```python
from build123d import *

# Parameters (mm, degrees)
SKETCH_1_R          = 2.2
SKETCH_1_R_2        = 1.95
SKETCH_1_W          = 40
SKETCH_1_H          = 20
SKETCH_1_W_2        = 16
EXTRUDE_1_DEPTH     = 1.5
SKETCH_2_W          = 120
SKETCH_2_H          = 3
EXTRUDE_2_DEPTH     = 6
SKETCH_3_R          = 2
CUT_EXTRUDE_1_DEPTH = 6


with BuildPart() as part:
    # 草图1 → 凸台-拉伸1 (new, symmetric)
    with BuildSketch(Plane.XY):
        Polygon((-0.084238348, 32.688738727), (91.943563532, 32.688738727), (91.943563532, -45.349139123), (-38.396296283, -45.349139123), (-38.396296283, -11.277844067), (-17.084238348, -11.277844067), (-0.084238348, -11.277844067), (-0.084238348, 8.722155933), align=None)
        with Locations((14.641461985, 3.722155933)):
            Circle(SKETCH_1_R, mode=Mode.SUBTRACT)
        with Locations((14.641461985, -6.277844067)):
            Circle(SKETCH_1_R, mode=Mode.SUBTRACT)
        with Locations((63.041461985, 3.722155933)):
            Circle(SKETCH_1_R, mode=Mode.SUBTRACT)
        with Locations((63.041461985, -6.277844067)):
            Circle(SKETCH_1_R, mode=Mode.SUBTRACT)
        with Locations((68.719491165, 27.139714958)):
            Circle(SKETCH_1_R_2, mode=Mode.SUBTRACT)
        with Locations((38.841461985, -1.277844067)):
            Rectangle(SKETCH_1_W, SKETCH_1_H, mode=Mode.SUBTRACT)
        with Locations((76.841461985, -1.277844067)):
            Rectangle(SKETCH_1_W_2, SKETCH_1_H, mode=Mode.SUBTRACT)
    extrude(amount=EXTRUDE_1_DEPTH, both=True)

    # 草图2 → 凸台-拉伸2 (add)
    with BuildSketch(Plane.XY.offset(1.5)):
        with Locations((21.603703717, -43.849139123)):
            Rectangle(SKETCH_2_W, SKETCH_2_H)
    extrude(amount=EXTRUDE_2_DEPTH)

    # 草图3 → 切除-拉伸1 (cut)
    with BuildSketch(Plane(origin=(0, -42.349139123, 0), x_dir=(1, 0, 0), z_dir=(0, 1, 0))):
        with Locations(Location((-31.396296283, -4.5, 0), (0, 0, 180))):
            Circle(SKETCH_3_R)
        with Locations(Location((74.603703717, -4.5, 0), (0, 0, 180))):
            Circle(SKETCH_3_R)
    extrude(amount=-CUT_EXTRUDE_1_DEPTH, mode=Mode.SUBTRACT)


solid = part.part
```
Work out the finished part from the listing and answer in its coordinate system (mm). A direction names the side the tool comes from. Round coordinates to 2 decimals unless told otherwise and drop trailing zeros. Write each loop counter-clockwise with the first axis right and the second up, starting at its lowest first coordinate (ties: lowest second). Pieces come first, ordered by that corner, then holes.
1) Which of the six approach directions +Z, -Z, +X, -X, +Y, -Y give full straight-line access (tool end or side, diameter ignored) to faces 4 (the face through (68.841, -1, 0)), 5 (the face through (-29.4, -43.8, 4.6)), 6 (the face through (81.604, -44, 4)), 7 (the face through (42, -14, -1.5)), 8 (the face through (21, -42.349, 4))?
2) A cutting plane is placed at A-A on z = 4.5. Determine the outline of the cut face in (x, y).
3) Consider probe 1 along Y at (x, z) = (27.5, 0.5); probe 2 along Y at (x, z) = (78, 4.75); probe 3 along Z at (x, y) = (-24, -38). Determine where each line is inside the solid, lowest interval first.
4) A cutting plane is placed at C-C on y = -14. Determine the outline of the cut face in (x, z), and give its area (3 significant figures).
5) A cutting plane is placed at B-B on x = -24. Determine the outline of the cut face in (y, z).
6) Flat-ended cylindrical pins translate along their axes: P1, Ø5, axis at x = 68.72, y = 27.14, coming from the +Z side; P2, Ø3.5, axis at x = -24.5, z = 0, coming from the +Y side; P3, Ø4.5, axis at x = -31.4, z = 4.5, coming from the +Y side. Find the tip coordinate at first contact, or state that the pin passes through.
7) Determine the mould class of faces 1 (the face through (21, -44, 7.5)), 2 (the face through (72.696, -43.828, 5.101)), 3 (the face through (-0.084, 11, 0)) for opening direction Z: pulls with the +Z half, pulls with the -Z half, needs draft (parallel to the pull), parting line crosses it, or undercut.
Entries:
1. face 4: +Z, -Z
1. face 5: +Y, -Y
1. face 6: +Z, +X, +Y, -Y
1. face 7: -Z, +X, -X, +Y, -Y
1. face 8: +Z, +X, -X, +Y
2. outline: (-38.4, -45.35) - (-33.4, -45.35) - (-33.4, -42.35) - (-38.4, -42.35) - close; (-29.4, -45.35) - (72.6, -45.35) - (72.6, -42.35) - (-29.4, -42.35) - close; (76.6, -45.35) - (81.6, -45.35) - (81.6, -42.35) - (76.6, -42.35) - close
3. probe 1: y = -45.35 to -11.28, 8.72 to 32.69
3. probe 2: y = -45.35 to -42.35
3. probe 3: z = -1.5 to 1.5
4. outline: (-38.4, -1.5) - (91.94, -1.5) - (91.94, 1.5) - (-38.4, 1.5) - close
4. area: 391 mm2
5. outline: (-45.35, -1.5) - (-11.28, -1.5) - (-11.28, 1.5) - (-42.35, 1.5) - (-42.35, 7.5) - (-45.35, 7.5) - close
6. P1: stops at z = 1.5
6. P2: stops at y = -11.28
6. P3: stops at y = -42.35
7. face 1: pulls with the +Z half
7. face 2: undercut
7. face 3: needs draft
